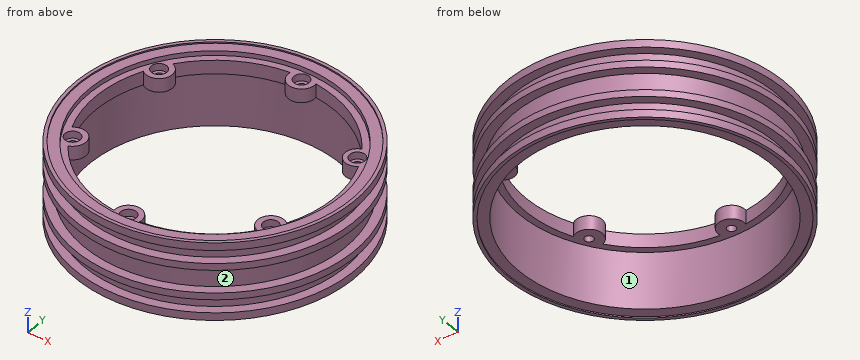
from build123d import *

# Parameters (mm, degrees)
ESTRUSIONE_ESTRUSIONE1_START = -4.15
SCHIZZO2_R                   = 38.135
SCHIZZO2_R_2                 = 1.3
ESTRUSIONE_ESTRUSIONE1_DEPTH = 4.15
SCHIZZO3_R                   = 2.325
TAGLIO_ESTRUSIONE1_DEPTH     = 2.15


with BuildPart() as part:
    # Schizzo1 → Rivoluzione1 (revolve)
    with BuildSketch(Plane(origin=(0, 0, 0), x_dir=(0, 0, -1), z_dir=(1, 0, 0)), mode=Mode.PRIVATE) as rivoluzione1_sk:
        Polygon((-11.41, 38.135), (11.41, 38.135), (11.41, 41.285), (11.81, 41.285), (11.81, 42.285), (9.49, 42.285), (9.49, 39.615), (5.52, 39.615), (5.52, 42.285), (3.44, 42.285), (3.44, 39.615), (-3.44, 39.615), (-3.44, 42.285), (-5.52, 42.285), (-5.52, 39.615), (-9.49, 39.615), (-9.49, 42.285), (-11.81, 42.285), (-11.81, 41.285), (-11.41, 41.285), align=None)
    revolve(rivoluzione1_sk.sketch.rotate(Axis((0, 0, 0), (0, 0, 1)), 90), axis=Axis((0, 0, 0), (0, 0, 1)))

    # Schizzo2 → Estrusione-Estrusione1 (add)
    with BuildSketch(Plane.XY.offset(10.01).offset(ESTRUSIONE_ESTRUSIONE1_START)):
        with Locations(Location((0, 0, 0), (0, 0, 180))):
            Circle(SCHIZZO2_R)
        with Locations((0, 35.25)):
            Circle(SCHIZZO2_R_2, mode=Mode.SUBTRACT)
        with Locations((30.527395483, 17.625)):
            Circle(SCHIZZO2_R_2, mode=Mode.SUBTRACT)
        with Locations((30.527395483, -17.625)):
            Circle(SCHIZZO2_R_2, mode=Mode.SUBTRACT)
        with Locations((0, -35.25)):
            Circle(SCHIZZO2_R_2, mode=Mode.SUBTRACT)
        with Locations((-30.527395483, -17.625)):
            Circle(SCHIZZO2_R_2, mode=Mode.SUBTRACT)
        with Locations((-30.527395483, 17.625)):
            Circle(SCHIZZO2_R_2, mode=Mode.SUBTRACT)
        with BuildLine():
            ThreePointArc((-33.078719897, 14.544294929), (-36.135, 0), (-33.078719897, -14.544294929))
            ThreePointArc((-33.078719897, -14.544294929), (-27.063293868, -15.625), (-29.135088837, -21.374864291))
            ThreePointArc((-29.135088837, -21.374864291), (-18.0675, -31.293827966), (-3.94363106, -35.91915922))
            ThreePointArc((-3.94363106, -35.91915922), (0, -31.25), (3.94363106, -35.91915922))
            ThreePointArc((3.94363106, -35.91915922), (18.0675, -31.293827966), (29.135088837, -21.374864291))
            ThreePointArc((29.135088837, -21.374864291), (27.063293868, -15.625), (33.078719897, -14.544294929))
            ThreePointArc((33.078719897, -14.544294929), (36.134649477, 0.159160806), (32.949313569, 14.835125895))
            ThreePointArc((32.949313569, 14.835125895), (27.327893405, 15.777766614), (29.322252678, 21.117379641))
            ThreePointArc((29.322252678, 21.117379641), (18.20516204, 31.213944001), (3.94363106, 35.91915922))
            ThreePointArc((3.94363106, 35.91915922), (0, 31.25), (-3.94363106, 35.91915922))
            ThreePointArc((-3.94363106, 35.91915922), (-18.0675, 31.293827966), (-29.135088837, 21.374864291))
            ThreePointArc((-29.135088837, 21.374864291), (-27.063293868, 15.625), (-33.078719897, 14.544294929))
        make_face(mode=Mode.SUBTRACT)
    extrude(amount=ESTRUSIONE_ESTRUSIONE1_DEPTH)

    # Schizzo3 → Taglio-Estrusione1 (cut)
    with BuildSketch(Plane(origin=(0, 0, 10.01), x_dir=(-1, 0, 0), z_dir=(0, 0, -1))):
        with Locations(Location((30.527395483, -17.625, 0), (0, 0, 180))):
            Circle(SCHIZZO3_R)
        with Locations(Location((0, -35.25, 0), (0, 0, 180))):
            Circle(SCHIZZO3_R)
        with Locations(Location((-30.527395483, -17.625, 0), (0, 0, 180))):
            Circle(SCHIZZO3_R)
        with Locations(Location((-30.527395483, 17.625, 0), (0, 0, 180))):
            Circle(SCHIZZO3_R)
        with Locations(Location((0, 35.25, 0), (0, 0, 180))):
            Circle(SCHIZZO3_R)
        with Locations(Location((30.527395483, 17.625, 0), (0, 0, 180))):
            Circle(SCHIZZO3_R)
    extrude(amount=TAGLIO_ESTRUSIONE1_DEPTH, mode=Mode.SUBTRACT)


solid = part.part
Geometry: final body of the model. Coordinates: model frame, mm. Face numbers are marked on the shaded views. Give positions to 0.01 mm unless a question says otherwise; leave off trailing zeros. Loops run counter-clockwise (first coordinate to the right, second up) from the corner with the lowest first, then second, coordinate; pieces in that order, holes last. Notation, with made-up numbers: (76, 65.25) - (100, 65.25) arc R34 ccw to (100, 100.25) - close; hole circle Ø8 at (18, 8.25). An arc over 180 degrees is marked (long way). Answer as CSV lines item,"result". Start each with the question number.
1. Section A-A, the plane x = 0. Give the number of separate pieces and of enclosed holes in the cut face, plus the area to 3 significant figures.
2. Section B-B, the plane z = 4.5. Return loops of the section in (x, y) (3 decimals), plus the area to 3 significant figures.
3. Pin query (flat end, axial travel): P1, Ø1.4, axis at x = 30, y = 17.5, coming from the +Z side; P2, Ø5, axis at y = 33.5, z = 4.5, coming from the +X side; P3, Ø12, axis at x = -21.5, y = 23, coming from the +Z side; P4, Ø1.5, axis at y = -28.5, z = 4.5, coming from the +X side. Return the tip coordinate at first contact, or that it passes through.
4. Section C-C, the plane z = -0.75. Return loops of the section in (x, y) (3 decimals).
5. Ray query, L1, parallel to Z at x = -19.5, y = 35.5; L2, parallel to X at y = -1, z = -2.25; L3, parallel to Z at x = 38.5, y = 17. Return the intervals inside material, ascending.
6. Draft query along X for the marked faces 1 and 2. Return one class per face: released by +X, released by -X, zero draft, split by the parting line, or undercut.
Answers:
1,separate pieces,"4"
1,enclosed holes,"0"
1,area,"139 mm2"
2,outline,"circle Ø84.57 at (0, 0); hole circle Ø76.27 at (0, 0)"
2,area,"1,050 mm2"
3,P1,"passes through"
3,P2,"stops at x = 28.76"
3,P3,"stops at z = 10.01"
3,P4,"stops at x = 31.91"
4,outline,"circle Ø79.23 at (0, 0); hole circle Ø76.27 at (0, 0)"
5,L1,"z = -11.41 to -9.49, -5.52 to -3.44, 3.44 to 5.52, 9.49 to 11.41"
5,L2,"x = -39.6 to -38.12, 38.12 to 39.6"
5,L3,"z = -11.81 to -9.49, -5.52 to -3.44, 3.44 to 5.52, 9.49 to 11.81"
6,face 1,"undercut"
6,face 2,"split by the parting line"
